```python
from build123d import *

# Parameters (mm, degrees)
SKETCH_1_W               = 20
SKETCH_1_H               = 20
EXTRUDE_1_DEPTH          = 31
SKETCH_4_R               = 2.7
CUT_EXTRUDE_3_DEPTH      = 9999
SKETCH_2_W               = 7.2
SKETCH_2_H               = 1.2
SKETCH_2_W_2             = 6.2
SKETCH_2_H_2             = 3.4
CUT_EXTRUDE_1_DEPTH      = 9999
CUT_EXTRUDE_2_DEPTH      = 9999
PATTERN_CIRCULAR_5_COUNT = 4
FILLET_1_R               = 1.5


with BuildPart() as part:
    # 草图1 → 凸台-拉伸1 (new, symmetric)
    with BuildSketch(Plane(origin=(0, 0, 0), x_dir=(1, 0, 0), z_dir=(0, 1, 0))):
        Rectangle(SKETCH_1_W, SKETCH_1_H)
    extrude(amount=EXTRUDE_1_DEPTH, both=True)

    # 草图4 → 切除-拉伸3 (cut)
    with BuildSketch(Plane(origin=(0, 31, 0), x_dir=(1, 0, 0), z_dir=(0, 1, 0))):
        with Locations(Location((0, 0, 0), (0, 0, 270))):
            Circle(SKETCH_4_R)
    extrude(amount=-CUT_EXTRUDE_3_DEPTH, mode=Mode.SUBTRACT)

    # 草图2 → 切除-拉伸1 (cut)
    with BuildSketch(Plane(origin=(0, 31, 0), x_dir=(1, 0, 0), z_dir=(0, 1, 0))):
        with Locations((0, 10)):
            Rectangle(SKETCH_2_W, SKETCH_2_H)
        with Locations((0, 10)):
            Rectangle(SKETCH_2_W_2, SKETCH_2_H_2)
    cut_extrude_1 = extrude(amount=-CUT_EXTRUDE_1_DEPTH, mode=Mode.SUBTRACT)

    # 草图3 → 切除-拉伸2 (cut)
    with BuildSketch(Plane(origin=(0, 31, 0), x_dir=(1, 0, 0), z_dir=(0, 1, 0))):
        Polygon((5.5, 8.3), (-5.5, 8.3), (-5.5, 6.3), (-3, 3.8), (3, 3.8), (5.5, 6.3), align=None)
    cut_extrude_2 = extrude(amount=-CUT_EXTRUDE_2_DEPTH, mode=Mode.SUBTRACT)

    # 阵列(圆周)5: 切除-拉伸1, 切除-拉伸2 ×4 about axis
    pattern_circular_5_axis = Axis((0, 0, 0), (0, 1, 0))
    add([cut_extrude_1.rotate(pattern_circular_5_axis, i * 360 / PATTERN_CIRCULAR_5_COUNT) for i in range(1, PATTERN_CIRCULAR_5_COUNT)], mode=Mode.SUBTRACT)
    add([cut_extrude_2.rotate(pattern_circular_5_axis, i * 360 / PATTERN_CIRCULAR_5_COUNT) for i in range(1, PATTERN_CIRCULAR_5_COUNT)], mode=Mode.SUBTRACT)

    # 圆角1
    fillet_1_edges = [part.edges().sort_by_distance(p)[0] for p in [
        (10, 0, 10),
        (-10, 0, 10),
        (-10, 0, -10),
        (10, 0, -10),
    ]]
    fillet(fillet_1_edges, radius=FILLET_1_R)


solid = part.part
```
Read the model definition and answer for the solid it produces. Units are mm, in the model's axes. A direction names the side the tool comes from. Coordinates: 2 decimals unless noted, no trailing zeros. Loops run counter-clockwise (first coordinate to the right, second up) from the corner with the lowest first, then second, coordinate; pieces in that order, holes last. Notation, with made-up numbers: (-28, -30.75) - (7, -30.75) arc R29 cw to (7, 4.25) - close; hole circle Ø5 at (46.25, 28). An arc over 180 degrees is marked (long way). Answer in a Markdown table with one row per item.
1. Find section B-B, the plane z = 0. Write down the section's boundary in (x, y), then the cut area to 3 significant figures.
Conclusion:
| item | result |
|---|---|
| outline | (-3.8, -31) - (-2.7, -31) - (-2.7, 31) - (-3.8, 31) - close; (2.7, -31) - (3.8, -31) - (3.8, 31) - (2.7, 31) - close |
| area | 136 mm² |
2. Determine the mould class of faces 5 (the face through (-6, 0, -10)), 6 (the face through (-7, 0, -5.5)), 7 (the face through (5, 0.4, 4.2)), 8 (the face through (3.8, 0, 0)) for opening direction X: +X half, -X half, draft (parallel to the pull), parting line (faces both ways), or undercut.
Conclusion:
| item | result |
|---|---|
| face 5 | draft |
| face 6 | undercut |
| face 7 | undercut |
| face 8 | +X half |
3. Which of the six approach directions +Z, -Z, +X, -X, +Y, -Y give full straight-line access (tool end or side, diameter ignored) to faces 1 (the face through (-9, 0, -3.1)), 2 (the face through (3.1, 0, -9)), 3 (the face through (-9.57, 0.43, 9.55)), 4 (the face through (-4.2, 0.4, 5))?
Conclusion:
| item | result |
|---|---|
| face 1 | -X, +Y, -Y |
| face 2 | -Z, +Y, -Y |
| face 3 | +Z, -X, +Y, -Y |
| face 4 | +Y, -Y |
4. Find section A-A, the plane x = -7. Write down the section's boundary in (y, z).
Conclusion:
| item | result |
|---|---|
| outline | (-31, -10) - (31, -10) - (31, -5.5) - (-31, -5.5) - close; (-31, 5.5) - (31, 5.5) - (31, 10) - (-31, 10) - close |
5. Given pin 1 (0.5 mm diameter, centred on y = 7.5, z = 10, fed in from +X); pin 2 (2 mm diameter, centred on x = -1.5, y = -22.5, fed in from +Z); pin 3 (1.8 mm diameter, centred on y = 3, z = 0.5, fed in from -X); pin 4 (4 mm diameter, centred on x = 6, z = -1.5, fed in from -Y), each flat-ended and moving along its own axis, determine where each tip first touches the part or whether it passes through.
Conclusion:
| item | result |
|---|---|
| pin 1 | stops at x = 9.33 |
| pin 2 | stops at z = 3.8 |
| pin 3 | stops at x = -3.8 |
| pin 4 | passes through |
6. Straight lines are drawn through the part: line 1 (X direction, y = 1.5, z = 0); line 2 (Z direction, x = 4.5, y = -25.5); line 3 (Z direction, x = 5, y = -6.5). For each, find the intervals that lie inside material, in ascending order.
Conclusion:
| item | result |
|---|---|
| line 1 | x = -3.8 to -2.7, 2.7 to 3.8 |
| line 2 | z = -10 to -8.3, -5.3 to -3.7, 3.7 to 5.3, 8.3 to 10 |
| line 3 | z = -10 to -8.3, -5.8 to -4.2, 4.2 to 5.8, 8.3 to 10 |
